Geometry: final body of the model. Coordinates: model frame, mm. A direction names the side the tool comes from. Round coordinates to 2 decimals unless told otherwise and drop trailing zeros. Write each loop counter-clockwise with the first axis right and the second up, starting at its lowest first coordinate (ties: lowest second). Pieces come first, ordered by that corner, then holes. Notation, with made-up numbers: M -29.75,57.5 L -20.75,57.5 A25 cw -20.75,70.5 Z; hole C 43.25,61 d4. An arc over 180 degrees is marked long. Use one line per item in the form item = value. Start each with the question number.
Item 1: Reachability of faces 4 (the flat face through (-19.1, -14, 1.5)), 5 (the flat face through (15.5, -14, 1.5)), 6 (the flat face through (-12, -69.633, 1)) from +Z, -Z, +X, -X, +Y, -Y: full face, straight path, thin tool, end or side. Return the list, or none.
Item 2: Pin query (flat end, axial travel): pin 1 Ø0.9 at (x, z) = (-13.5, 1) entering from +Y; pin 2 Ø1 at (x, z) = (15, 0.5) entering from +Y. Return the tip coordinate at first contact, or that it passes through.
Item 3: Section query A-A (y = -23.75). Return loops of the section in (x, z).
Item 4: Section query D-D (x = 13.5). Return loops of the section in (y, z).
Item 5: Section query C-C (x = -5.1). Return loops of the section in (y, z), and give its area (3 significant figures).
Item 6: Pull-direction query (X, two-part tool) for faces 1 (the flat face through (-5, -90.456, 2)), 2 (the flat face through (-15.5, -14, 1.5)), 3 (the flat face through (-20.1, -49, 2)); classes: pulls with the +X half, pulls with the -X half, needs draft (parallel to the pull), parting line crosses it, or undercut.
Item 7: Ray query, probe 1 along Y at (x, z) = (-5.1, 1.2); probe 2 along X at (y, z) = (-77.5, 1.8); probe 3 along X at (y, z) = (-21, 2). Return the intervals inside material, ascending.
Item 8: Section query B-B (y = -45). Return loops of the section in (x, z), and give its area (3 significant figures).
from build123d import *

# Parameters (mm, degrees)
IZIM1_R                     = 2.1
IZIM1_R_2                   = 1.6
Y_KSEKLIK_EKSTR_ZYON1_DEPTH = 3
Y_KSEKLIK_EKSTR_ZYON2_DEPTH = 3
IZIM5_R                     = 1.5
KES_EKSTR_ZYON1_DEPTH       = 4
SKETCH3_W                   = 8
SKETCH3_H                   = 20
CUT_EXTRUDE1_DEPTH          = 10


with BuildPart() as part:
    # Çizim1 → Yükseklik-Ekstrüzyon1 (new body)
    with BuildSketch(Plane.XY.offset(3)):
        with BuildLine():
            Line((-20.1, -15), (-20.1, -83.384802))
            Line((-20.1, -83.384802), (-13.028932188, -90.455869812))
            Line((-13.028932188, -90.455869812), (3.075751729, -90.455869812))
            Line((3.075751729, -90.455869812), (10.146819541, -83.384802))
            Line((10.146819541, -83.384802), (10.146819541, -73.586547015))
            Line((10.146819541, -73.586547015), (19.709913851, -64.023452705))
            Line((19.709913851, -64.023452705), (19.709913851, -14.740055992))
            Line((19.709913851, -14.740055992), (18.1, -13))
            Line((18.1, -13), (16.5, -13))
            Line((16.5, -13), (14.5, -15))
            Line((14.5, -15), (14.5, -41.5))
            ThreePointArc((14.5, -41.5), (14.207106781, -42.207106781), (13.5, -42.5))
            Line((13.5, -42.5), (-13.5, -42.5))
            ThreePointArc((-13.5, -42.5), (-14.207106781, -42.207106781), (-14.5, -41.5))
            Line((-14.5, -41.5), (-14.5, -15))
            Line((-14.5, -15), (-16.5, -13))
            Line((-16.5, -13), (-18.1, -13))
            Line((-18.1, -13), (-20.1, -15))
        make_face()
        with Locations((-5.1, -77.455869812)):
            Circle(IZIM1_R, mode=Mode.SUBTRACT)
        with Locations((-5.1, -85.455869812)):
            Circle(IZIM1_R_2, mode=Mode.SUBTRACT)
    extrude(amount=-Y_KSEKLIK_EKSTR_ZYON1_DEPTH)

    # Çizim4 → Yükseklik-Ekstrüzyon2 (add)
    with BuildSketch(Plane.XY.offset(3)):
        Polygon((-16.5, -13), (-14.5, -15), (-11, -15), (-11, -42.5), (11, -42.5), (11, -15), (14.5, -15), (16.5, -13), (16.5, -43.147363563), (-16.5, -43.147363563), align=None)
    extrude(amount=-Y_KSEKLIK_EKSTR_ZYON2_DEPTH)

    # Çizim5 → Kes-Ekstrüzyon1 (cut)
    with BuildSketch(Plane(origin=(0, 0, 0), x_dir=(-1, 0, 0), z_dir=(0, 0, -1))):
        with Locations((-13.5, -23.75)):
            Circle(IZIM5_R)
        with Locations((-13.5, -31.75)):
            Circle(IZIM5_R)
        with Locations((-13.5, -39.75)):
            Circle(IZIM5_R)
        with Locations((-7.609913851, -45)):
            Circle(IZIM5_R)
        with Locations((8, -45)):
            Circle(IZIM5_R)
        with Locations((13.5, -39.75)):
            Circle(IZIM5_R)
        with Locations((13.5, -31.75)):
            Circle(IZIM5_R)
        with Locations((13.5, -23.75)):
            Circle(IZIM5_R)
    extrude(amount=-KES_EKSTR_ZYON1_DEPTH, mode=Mode.SUBTRACT)

    # Sketch3 → Cut-Extrude1 (cut)
    with BuildSketch(Plane(origin=(0, 0, 0), x_dir=(-1, 0, 0), z_dir=(0, 0, -1))):
        with Locations((12.1, -59.633395866)):
            Rectangle(SKETCH3_W, SKETCH3_H)
        Polygon((-15.709913851, -49.633395866), (-15.709913851, -61.633395866), (-7.709913851, -69.633395866), (-7.709913851, -49.633395866), align=None)
    extrude(amount=-CUT_EXTRUDE1_DEPTH, mode=Mode.SUBTRACT)


solid = part.part
Working result:
q1.face_4 = +Z, -Z, -X, +Y
q1.face_5 = +Z, -Z, +Y
q1.face_6 = +Z, -Z
q2.pin_1 = -15
q2.pin_2 = -14
q3.outline = M -20.1,0 L -15,0 L -15,3 L -20.1,3 Z; M -12,0 L -11,0 L -11,3 L -12,3 Z; M 11,0 L 12,0 L 12,3 L 11,3 Z; M 15,0 L 19.71,0 L 19.71,3 L 15,3 Z
q4.outline = M -70.23,0 L -63.84,0 L -63.84,3 L -70.23,3 Z; M -49.63,0 L -41.25,0 L -41.25,3 L -49.63,3 Z; M -38.25,0 L -33.25,0 L -33.25,3 L -38.25,3 Z; M -30.25,0 L -25.25,0 L -25.25,3 L -30.25,3 Z; M -22.25,0 L -15,0 L -15,3 L -22.25,3 Z
q5.outline = M -90.46,0 L -87.06,0 L -87.06,3 L -90.46,3 Z; M -83.86,0 L -79.56,0 L -79.56,3 L -83.86,3 Z; M -75.36,0 L -42.5,0 L -42.5,3 L -75.36,3 Z
q5.area = 122 mm²
q6.face_1 = needs draft
q6.face_2 = undercut
q6.face_3 = pulls with the -X half
q7.probe_1 = -90.46 to -87.06, -83.86 to -79.56, -75.36 to -42.5
q7.probe_2 = -20.1 to -7.2, -3 to 10.15
q7.probe_3 = -20.1 to -11, 11 to 19.71
q8.outline = M -20.1,0 L -9.5,0 L -9.5,3 L -20.1,3 Z; M -6.5,0 L 6.11,0 L 6.11,3 L -6.5,3 Z; M 9.11,0 L 19.71,0 L 19.71,3 L 9.11,3 Z
q8.area = 101 mm²
